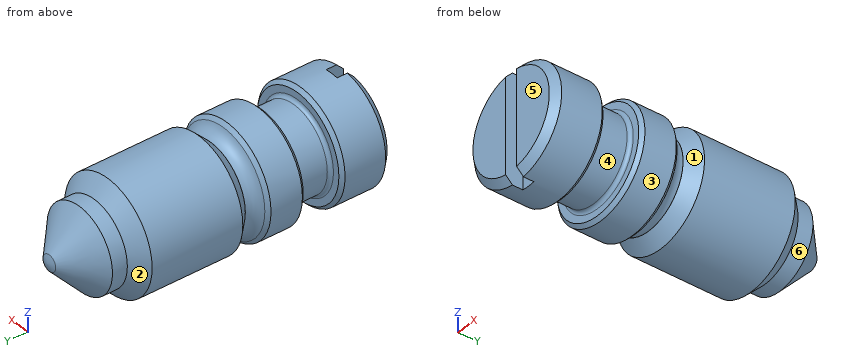
from build123d import *

# Parameters (mm, degrees)
REDONDEO1_R           = 0.25
CHAFL_N7_SIZE         = 0.25
CHAFL_N9_SIZE         = 0.5
CROQUIS1_W            = 1
CROQUIS1_H            = 1.25
CORTAR_EXTRUIR1_DEPTH = 40
REDONDEO2_R           = 1


with BuildPart() as part:
    # Sketch1 → Revolve1 (revolve)
    with BuildSketch(Plane.XY):
        with BuildLine():
            Line((0, 0), (-3.99720796, 0))
            Line((-3.99720796, 0), (-3.99720796, 3.695721343))
            Line((-3.99720796, 3.695721343), (-3, 3.695721343))
            Line((-3, 3.695721343), (-3, 6.290801943))
            Line((-3, 6.290801943), (-3.996490616, 6.290801943))
            Line((-3.996490616, 6.290801943), (-3.996490616, 9.069605063))
            Line((-3.996490616, 9.069605063), (-3.13, 9.069605063))
            Line((-3.13, 9.069605063), (-3.13, 10))
            Line((-3.13, 10), (-3.997062109, 10.867062109))
            Line((-3.997062109, 10.867062109), (-3.997062109, 17.446452736))
            Line((-3.997062109, 17.446452736), (-2.993514845, 18.45))
            Line((-2.993514845, 18.45), (-2.993514845, 19.528543236))
            Line((-2.993514845, 19.528543236), (-0.584226233, 21.734587674))
            ThreePointArc((-0.584226233, 21.734587674), (-0.297614848, 21.830829517), (0, 21.884064665))
            Line((0, 21.884064665), (0, 0))
        make_face()
    revolve(axis=Axis((0, 21.884064665, 0), (0, -1, 0)))

    # Redondeo1
    redondeo1_edges = [part.edges().sort_by_distance(p)[0] for p in [
        (3, 6.290801943, 0),
        (3, 3.695721343, 0),
    ]]
    fillet(redondeo1_edges, radius=REDONDEO1_R)

    # Chaflán7
    chafl_n7_edges = [part.edges().sort_by_distance(p)[0] for p in [
        (3.996490616, 9.069605063, 0),
        (3.996490616, 6.290801943, 0),
        (3.99720796, 3.695721343, 0),
    ]]
    chamfer(chafl_n7_edges, length=CHAFL_N7_SIZE)

    # Chaflán9
    chafl_n9_edges = [part.edges().sort_by_distance(p)[0] for p in [
        (3.99720796, 0, 0),
    ]]
    chamfer(chafl_n9_edges, length=CHAFL_N9_SIZE)

    # Croquis1 → Cortar-Extruir1 (cut)
    with BuildSketch(Plane.XY.offset(10)):
        with Locations((0, 0.625)):
            Rectangle(CROQUIS1_W, CROQUIS1_H)
    extrude(amount=-CORTAR_EXTRUIR1_DEPTH, mode=Mode.SUBTRACT)

    # Redondeo2
    # the kernel refuses this fillet: 1 mm, written as the material it adds along each edge
    with BuildSketch(Plane(origin=(0, 9.069605063, 0), x_dir=(-1, 0, 0), z_dir=(0, 0, 1))) as redondeo2_piece_1:
        with BuildLine():
            CenterArc((4.13, -0.923536979), REDONDEO2_R, 112.55123215, 67.44876785)
            Line((3.13, -0.923536979), (3.11, -0.923536979))
            Line((3.11, -0.923536979), (3.11, 0))
            Line((3.11, 0), (3.13, 0.02))
            ThreePointArc((3.13, 0.02), (3.438245308, 0.02), (3.738820428, 0.01847074))
            Line((3.738820428, 0.01847074), (3.746490616, 0))
        make_face()
    revolve(axis=Axis((0, 9.069605063, 0), (0, -1, 0)))


solid = part.part
Source: CAD feature listing. Evaluate the final solid. Frame: model axes, mm. Face numbers are marked on the shaded views. A direction names the side the tool comes from. Give positions to 0.01 mm unless a question says otherwise; leave off trailing zeros. Order: outer loops, then holes, each group sorted by start corner. A loop starts at its lowest first (then second) coordinate and runs counter-clockwise, first axis right, second up. Notation, with made-up numbers: (7, -16.5) -> (33, -16.5) arc R31 cw to (33, 8.5) -> close; hole circle Ø10 at (13, 82). An arc over 180 degrees is marked (long way). Write item = value, one per line.
Item 1: Set-up query: the marked faces 5 and 6. Return all of +Z, -Z, +X, -X, +Y, -Y with unobstructed straight access to the full face (end or side cutting, diameter ignored); none if empty.
Check result:
face_5 = +Z, -Z, +X, -X, -Y
face_6 = +Y
Item 2: Contact query for flat-ended pins moving along their axis: pin 1 (1.5 mm diameter, centred on y = 8.5, z = 3, fed in from +X); pin 2 (3 mm diameter, centred on x = 2.5, z = -2, fed in from +Y); pin 3 (1.5 mm diameter, centred on y = 12.5, z = -1, fed in from +X). Output: stop coordinate, or through.
Check result:
pin_1 = 3.3
pin_2 = 20.71
pin_3 = 3.99
Item 3: Ray query, probe 1 along Y at (x, z) = (-2.75, 2.75); probe 2 along Y at (x, z) = (-3.25, -1); probe 3 along Z at (x, y) = (-2, 16). Return the intervals inside material, ascending.
Check result:
probe_1 = 0.39 to 3.55, 6.43 to 8.93, 10.76 to 17.55
probe_2 = 0 to 3.7, 6.29 to 9.31, 10.27 to 18.04
probe_3 = -3.46 to 3.46
Item 4: Mould query, pull axis Y, two halves, no side actions, for the marked faces 1, 2, 3 and 4. Classes: +Y half, -Y half, draft (parallel to the pull), parting line (faces both ways), or undercut.
Check result:
face_1 = undercut
face_2 = +Y half
face_3 = draft
face_4 = undercut
Item 5: Section query A-A (y = 10.5). Output: boundary loops of the cut face in (x, z).
Check result:
outline = circle Ø7.26 at (0, 0)
Item 6: Section query B-B (y = 15). Output: boundary loops of the cut face in (x, z), then the cut area to 3 significant figures.
Check result:
outline = circle Ø7.99 at (0, 0)
area = 50.2 mm²
